The listing builds one solid part. Answer for the finished solid, in the listing's coordinates (mm). Face numbers are marked on the shaded views. A direction names the side the tool comes from. Coordinates: 2 decimals unless noted, no trailing zeros. Write each loop counter-clockwise with the first axis right and the second up, starting at its lowest first coordinate (ties: lowest second). Pieces come first, ordered by that corner, then holes.
from build123d import *

# Parameters (mm, degrees)
F1_DEPTH      = 12.5
F3_DEPTH      = 9
F4_W          = 10
F4_H          = 5
F6_R          = 3
F7_R          = 1.5
F8_DEPTH      = 12.5010001
F8_DEPTH_BACK = 12.5010001
F9_W          = 4
F9_H          = 20
F10_DEPTH     = 2
F11_R         = 0.7
F12_R         = 15


with BuildPart() as f1:
    # F0 (on Front) → F1 (new body, symmetric)
    with BuildSketch(Plane.XZ):
        with BuildLine():
            Line((-35.5, 7.5), (-12.409673646, 7.5))
            ThreePointArc((-12.409673646, 7.5), (7.1239034244, -12.6293309403), (0, 14.5))
            Line((0, 14.5), (-35.5, 14.5))
            Line((-35.5, 14.5), (-35.5, 7.5))
        make_face()
    extrude(amount=F1_DEPTH, both=True)

    # F2 (on Front) → F3 (cut, symmetric)
    with BuildSketch(Plane.XZ):
        with BuildLine():
            Line((-10.5897720282, 11.5), (-10.5897720282, 6.6412896632))
            ThreePointArc((-10.5897720282, 6.6412896632), (7.0386819061, -10.3299059543), (-2.3066189308, 12.2853371589))
            Line((-2.3066189308, 12.2853371589), (1.4102279718, 14.4312597187))
            ThreePointArc((1.4102279718, 14.4312597187), (0.7059511596, 14.4828047339), (0, 14.5))
            Line((0, 14.5), (-10.5897720282, 14.5))
            Line((-10.5897720282, 14.5), (-10.5897720282, 12.5))
            Line((-10.5897720282, 12.5), (-35.5, 12.5))
            Line((-35.5, 12.5), (-35.5, 9))
            Line((-35.5, 9), (-10.5897720282, 11.5))
        make_face()
    extrude(amount=F3_DEPTH, both=True, mode=Mode.SUBTRACT)

    # F4 (on Front) → F5 (revolve)
    with BuildSketch(Plane.XZ):
        with Locations((17.5, 2.5)):
            Rectangle(F4_W, F4_H)
    revolve(axis=Axis((17.5, 0, 0), (-1, 0, 0)))

    # F6
    f6_edges = [f1.edges().sort_by_distance(p)[0] for p in [
        (22.5, 0, -5),
    ]]
    fillet(f6_edges, radius=F6_R)

    # F7 (on Front) → F8 (cut, two sides)
    with BuildSketch(Plane.XZ) as f8_sk:
        with Locations((17.5, 0)):
            Circle(F7_R)
    extrude(amount=-F8_DEPTH, mode=Mode.SUBTRACT)
    extrude(f8_sk.sketch, amount=F8_DEPTH_BACK, mode=Mode.SUBTRACT)

    # F9 (on face) → F10 (join)
    with BuildSketch(Plane(origin=(0, 0, 7.5), x_dir=(1, 0, 0), z_dir=(0, 0, -1))):
        with Locations((-33.5, 0)):
            Rectangle(F9_W, F9_H)
    extrude(amount=F10_DEPTH)

    # F11
    f11_edges = [f1.edges().sort_by_distance(p)[0] for p in [
        (-33.5, -10, 7.5),
        (-31.5, 0, 7.5),
        (-33.5, 10, 7.5),
        (-33.5, 10, 5.5),
        (-31.5, 0, 5.5),
        (-33.5, -10, 5.5),
        (-31.5, 10, 6.5),
        (-31.5, -10, 6.5),
    ]]
    fillet(f11_edges, radius=F11_R)

    # F12
    f12_edges = [f1.edges().sort_by_distance(p)[0] for p in [
        (-12.409674, 0, 7.5),
    ]]
    fillet(f12_edges, radius=F12_R)

    # F13 (on Front) → F14 (revolve)
    with BuildSketch(Plane.XZ):
        with BuildLine():
            Line((0, -12.6), (0, -1.6))
            ThreePointArc((0, -1.6), (-5.5, -7.1), (0, -12.6))
        make_face()
    revolve(axis=Axis((0, 0, -7.1), (0, 0, -1)))


solid = f1.part
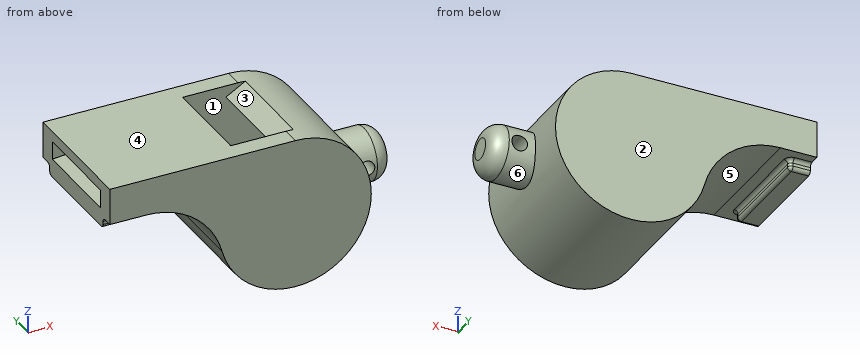
Q1. Determine the mould class of the marked faces 1, 2 and 3 for opening direction Z: released by +Z, released by -Z, zero draft, split by the parting line, or undercut.
Answers below:
face 1: undercut
face 2: zero draft
face 3: released by +Z
Q2. Find the intervals of material crossed by probe 1 along X at (y, z) = (4, -7.75); probe 2 along Y at (x, z) = (-2.5, 8); probe 3 along Z at (x, y) = (0, -2.25), in increasing order.
Answers below:
probe 1: x = -12.26 to -9.81, -3.72 to 3.72, 9.81 to 12.26
probe 2: y = -12.5 to -9, 9 to 12.5
probe 3: z = -14.5 to -12.5, -12.12 to -2.08, 12.5 to 13.62
Q3. The part is cut by section A-A, the plane y = 6.5. Write down the section's boundary in (x, z), then the cut area to 3 significant figures.
Answers below:
outline: (-35.5, 5.5) - (-32.2, 5.5) arc R0.7 ccw to (-31.5, 6.2) - (-31.5, 6.8) arc R0.7 cw to (-30.8, 7.5) - (-28.53, 7.5) arc R15 cw to (-14.02, -3.69) arc R14.5 ccw (long way) to (1.41, 14.43) - (-2.31, 12.29) arc R12.5 cw (long way) to (-10.59, 6.64) - (-10.59, 11.5) - (-35.5, 9) - close; (-35.5, 12.5) - (-10.59, 12.5) - (-10.59, 14.5) - (-35.5, 14.5) - close
area: 312 mm2
Q4. The part is cut by section C-C, the plane z = 8.25. Write down the section's boundary in (x, y).
Answers below:
outline: (-35.5, -12.5) - (11.92, -12.5) - (11.92, 12.5) - (-35.5, 12.5) - close; hole (-10.59, -9) - (9.39, -9) - (9.39, 9) - (-10.59, 9) - close
Q5. The part is cut by section B-B, the plane x = 9.5. Write down the section's boundary in (y, z), then the cut area to 3 significant figures.
Answers below:
outline: (-12.5, -10.95) - (12.5, -10.95) - (12.5, 10.95) - (-12.5, 10.95) - close; hole (-9, -8.12) - (9, -8.12) - (9, 8.12) - (-9, 8.12) - close
area: 255 mm2
Q6. Which of the six approach directions +Z, -Z, +X, -X, +Y, -Y give full straight-line access (tool end or side, diameter ignored) to the marked faces 4, 5 and 6?
Answers below:
face 4: +Z, +X, -X, +Y, -Y
face 5: -Z, +Y, -Y
face 6: +X
Q7. Given pin 1 (2.5 mm diameter, centred on y = 0, z = 9, fed in from +X); pin 2 (9 mm diameter, centred on x = -21, y = -0.5, fed in from -Z); pin 3 (5 mm diameter, centred on x = -20, y = -2.5, fed in from -Z), each flat-ended and moving along its own axis, determine where each tip first touches the part or whether it passes through.
Answers below:
pin 1: stops at x = 12.26
pin 2: stops at z = 1.46
pin 3: stops at z = 2.66
Q8. The part is cut by section D-D, the plane y = 0. State how many separate pieces and enclosed holes the cut face has, then the cut area to 3 significant figures.
Answers below:
separate pieces: 2
enclosed holes: 1
area: 479 mm2
